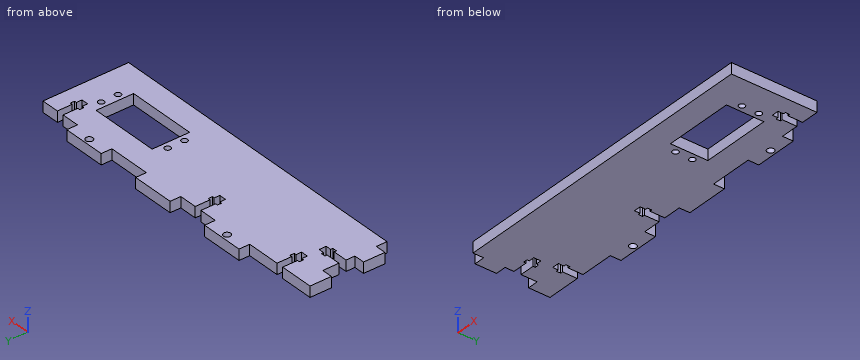
```python
from build123d import *

# Parameters (mm, degrees)
SKETCH1_W           = 190.5
SKETCH1_H           = 50.8
BOSS_EXTRUDE1_DEPTH = 6.35
SKETCH2_W           = 41.275
SKETCH2_H           = 22.225
CUT_EXTRUDE1_DEPTH  = 151.724377554
SKETCH3_W           = 25.4
SKETCH3_H           = 6.35
BOSS_EXTRUDE2_DEPTH = 6.35
LPATTERN1_COUNT     = 3
LPATTERN1_PITCH     = 50.8
SKETCH4_W           = 6.35
SKETCH4_H           = 12.7
BOSS_EXTRUDE3_DEPTH = 6.35
LPATTERN2_COUNT     = 2
LPATTERN2_PITCH     = 31.75
CUT_EXTRUDE2_DEPTH  = 6.35
SKETCH6_R           = 2.0955
CUT_EXTRUDE3_DEPTH  = 159.133368044
CUT_EXTRUDE4_DEPTH  = 159.133368044
SKETCH8_R           = 1.778
CUT_EXTRUDE5_DEPTH  = 159.133368044


with BuildPart() as part:
    # Sketch1 → Boss-Extrude1 (new body)
    with BuildSketch(Plane.XY):
        with Locations((-53.183, 0)):
            Rectangle(SKETCH1_W, SKETCH1_H)
    extrude(amount=BOSS_EXTRUDE1_DEPTH)

    # Sketch2 → Cut-Extrude1 (cut, through all)
    with BuildSketch(Plane.XY.offset(6.35)):
        Rectangle(SKETCH2_W, SKETCH2_H)
    extrude(amount=-CUT_EXTRUDE1_DEPTH, mode=Mode.SUBTRACT)

    # Sketch3 → Boss-Extrude2 (add)
    with BuildSketch(Plane(origin=(0, 25.4, 0), x_dir=(1, 0, 0), z_dir=(0, 1, 0))):
        with Locations((3.967, -3.175)):
            Rectangle(SKETCH3_W, SKETCH3_H)
    boss_extrude2 = extrude(amount=BOSS_EXTRUDE2_DEPTH)

    # LPattern1: Boss-Extrude2 ×3
    with Locations(*[(-i * LPATTERN1_PITCH, 0, 0) for i in range(1, LPATTERN1_COUNT)]):
        add(boss_extrude2)

    # Sketch4 → Boss-Extrude3 (add)
    with BuildSketch(Plane.ZY.offset(148.433)):
        with Locations((3.175, 19.05)):
            Rectangle(SKETCH4_W, SKETCH4_H)
    boss_extrude3 = extrude(amount=BOSS_EXTRUDE3_DEPTH)

    # LPattern2: Boss-Extrude3 ×2
    with Locations(*[(0, -i * LPATTERN2_PITCH, 0) for i in range(1, LPATTERN2_COUNT)]):
        add(boss_extrude3)

    # Sketch5 → Cut-Extrude2 (cut)
    with BuildSketch(Plane.XY.offset(6.35)):
        Polygon((31.4625, 25.4), (27.2715, 25.4), (27.2715, 16.637), (25.938, 16.637), (25.938, 14.097), (27.2715, 14.097), (27.2715, 10.795), (31.4625, 10.795), (31.4625, 14.097), (32.796, 14.097), (32.796, 16.637), (31.4625, 16.637), align=None)
        Polygon((-70.1375, 25.4), (-74.3285, 25.4), (-74.3285, 16.637), (-75.662, 16.637), (-75.662, 14.097), (-74.3285, 14.097), (-74.3285, 10.795), (-70.1375, 10.795), (-70.1375, 14.097), (-68.804, 14.097), (-68.804, 16.637), (-70.1375, 16.637), align=None)
        Polygon((-130.4625, 25.4), (-134.6535, 25.4), (-134.6535, 16.637), (-135.987, 16.637), (-135.987, 14.097), (-134.6535, 14.097), (-134.6535, 10.795), (-130.4625, 10.795), (-130.4625, 14.097), (-129.129, 14.097), (-129.129, 16.637), (-130.4625, 16.637), align=None)
    extrude(amount=-CUT_EXTRUDE2_DEPTH, mode=Mode.SUBTRACT)

    # Sketch6 → Cut-Extrude3 (cut, through all)
    with BuildSketch(Plane(origin=(0, 0, 0), x_dir=(-1, 0, 0), z_dir=(0, 0, -1))):
        with Locations((-3.98760291, 28.575)):
            Circle(SKETCH6_R)
        with Locations((97.61239709, 28.575)):
            Circle(SKETCH6_R)
    extrude(amount=-CUT_EXTRUDE3_DEPTH, mode=Mode.SUBTRACT)

    # Sketch7 → Cut-Extrude4 (cut, through all)
    with BuildSketch(Plane.XY.offset(6.35)):
        Polygon((-148.433, 3.1115), (-148.433, -1.0795), (-139.67, -1.0795), (-139.67, -2.413), (-137.13, -2.413), (-137.13, -1.0795), (-133.828, -1.0795), (-133.828, 3.1115), (-137.13, 3.1115), (-137.13, 4.445), (-139.67, 4.445), (-139.67, 3.1115), align=None)
    extrude(amount=-CUT_EXTRUDE4_DEPTH, mode=Mode.SUBTRACT)

    # Sketch8 → Cut-Extrude5 (cut, through all)
    with BuildSketch(Plane(origin=(0, 0, 0), x_dir=(-1, 0, 0), z_dir=(0, 0, -1))):
        with Locations((24.5, -5)):
            Circle(SKETCH8_R)
        with Locations((24.5, 5)):
            Circle(SKETCH8_R)
        with Locations((-24.5, 5)):
            Circle(SKETCH8_R)
        with Locations((-24.5, -5)):
            Circle(SKETCH8_R)
    extrude(amount=-CUT_EXTRUDE5_DEPTH, mode=Mode.SUBTRACT)


solid = part.part
```
Part model, mm, in its own coordinate system. Give positions to 0.01 mm unless a question says otherwise; leave off trailing zeros. Write each loop counter-clockwise with the first axis right and the second up, starting at its lowest first coordinate (ties: lowest second). Pieces come first, ordered by that corner, then holes. Notation, with made-up numbers: (3.25, 34) -> (44.25, 34) arc R24 ccw to (44.25, 69) -> close; hole circle Ø5 at (11.5, 58). An arc over 180 degrees is marked (long way). Put each result on its own line as item: value. Start each with the question number.
Item 1: Cut at D-D (x = -66). List the corners of the cut face in (y, z).
Item 2: Cut at A-A (y = 22). List the corners of the cut face in (x, z).
Item 3: Pin check, flat tips, straight feed: pin 1 Ø2 at (x, z) = (-72.5, 3) entering from +Y (3 decimals); pin 2 Ø1.9 at (x, z) = (22.5, 4.5) entering from +Y; pin 3 Ø3 at (x, z) = (-151, 2) entering from -Y. Stop position of each tip, or through.
Item 4: Cut at B-B (x = -24.5). List the corners of the cut face in (y, z).
Item 5: Cut at C-C (z = 5.25). State how many separate pieces and enclosed holes the cut face has, then the cut area to 3 significant figures.
Item 6: Wall check: L1, parallel to Y at x = -24.5, z = 3.75; L2, parallel to X at y = 26, z = 3.5; L3, parallel to X at y = 29, z = 5. Give the ranges that are in metal, low to high. Write a range as [from, to].
Answer list:
1. outline: (-25.4, 0) -> (25.4, 0) -> (25.4, 6.35) -> (-25.4, 6.35) -> close
2. outline: (-154.78, 0) -> (-134.65, 0) -> (-134.65, 6.35) -> (-154.78, 6.35) -> close; (-130.46, 0) -> (-74.33, 0) -> (-74.33, 6.35) -> (-130.46, 6.35) -> close; (-70.14, 0) -> (27.27, 0) -> (27.27, 6.35) -> (-70.14, 6.35) -> close; (31.46, 0) -> (42.07, 0) -> (42.07, 6.35) -> (31.46, 6.35) -> close
3. pin 1: stops at y = 10.795
3. pin 2: stops at y = 25.4
3. pin 3: stops at y = -19.05
4. outline: (-25.4, 0) -> (-6.78, 0) -> (-6.78, 6.35) -> (-25.4, 6.35) -> close; (-3.22, 0) -> (3.22, 0) -> (3.22, 6.35) -> (-3.22, 6.35) -> close; (6.78, 0) -> (25.4, 0) -> (25.4, 6.35) -> (6.78, 6.35) -> close
5. separate pieces: 1
5. enclosed holes: 7
5. area: 9,070 mm2
6. L1: y = [-25.4, -6.78], [-3.22, 3.22], [6.78, 25.4]
6. L2: x = [-110.33, -84.93], [-59.53, -34.13], [-8.73, 16.67]
6. L3: x = [-110.33, -99.66], [-95.56, -84.93], [-59.53, -34.13], [-8.73, 1.94], [6.04, 16.67]
